Read the model definition and answer for the solid it produces. Units are mm, in the model's axes. Face numbers are marked on the shaded views. Coordinates: 2 decimals unless noted, no trailing zeros. Write each loop counter-clockwise with the first axis right and the second up, starting at its lowest first coordinate (ties: lowest second). Pieces come first, ordered by that corner, then holes. Notation, with made-up numbers: (-32, 34.25) -> (-1, 34.25) arc R24 cw to (-1, 59.25) -> close; hole circle Ø5 at (32.25, 56). An arc over 180 degrees is marked (long way). One line per item, written item: value. Start each with the question number.
1. Consider line 1 along Y through (x, z) = (14.5, 40.5); line 2 along Y through (x, z) = (-51, 8.5); line 3 along X through (y, z) = (-15, 31.5). Determine where each line is inside the solid, lowest interval first.
2. Find section B-B, the plane z = 34.5. Write down the section's boundary in (x, y), and give its area (3 significant figures).
3. Find section C-C, the plane x = -39. Write down the section's boundary in (y, z).
4. Given P1, Ø4, axis at y = -27, z = 23.5, coming from the +X side; P2, Ø9.5, axis at x = -85, y = -45, coming from the +Z side; P3, Ø4, axis at x = -6.5, y = 28.5, coming from the +Z side; P4, Ø4.5, axis at x = 14.47, y = -76.39, coming from the -Z side, each flat-ended and moving along its own axis, determine where each tip first touches the part or whether it passes through.
5. Find section D-D, the plane y = -62.5. Write down the section's boundary in (x, z), and give its area (3 significant figures).
6. For a pull along X with two mould halves and no side action, classify the marked faces 1, 2 and 3 as pulls with the +X half, pulls with the -X half, needs draft (parallel to the pull), parting line crosses it, or undercut.
7. Find section A-A, the plane z = 19. Write down the section's boundary in (x, y).
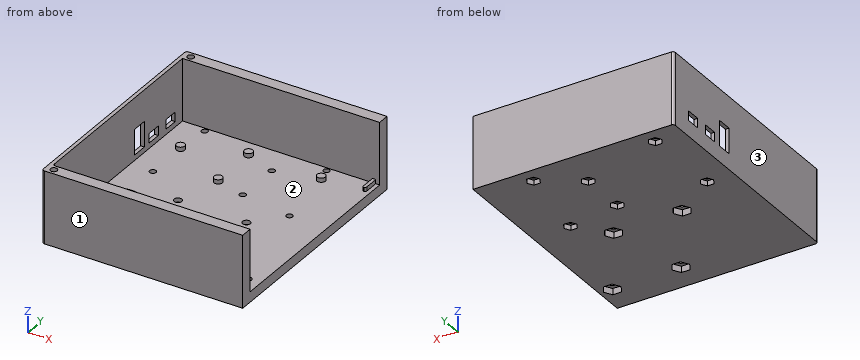
```python
from build123d import *

# Parameters (mm, degrees)
F5_W         = 192.786
F5_H         = 141.3764
F7_DEPTH     = 44.45
F12_W        = 187.452
F12_H        = 127
F14_DEPTH    = 38.1
F4_R         = 15.621
F4_R_2       = 13.081
F13_W        = 2.032
F13_H        = 10.16
F13_W_2      = 10.16
F13_H_2      = 2.032
F15_DEPTH    = 8.89
F16_DEPTH    = 2.9972
F17_DEPTH    = 3.81
F10_R        = 2.3749
F18_DEPTH    = 25.4
F3_R         = 1.9304
F19_DEPTH    = 25.4
F11_R        = 2.54
F20_DEPTH    = 8.89
F21_W        = 8.89
F21_H        = 5.842
F21_W_2      = 9.525
F21_H_2      = 15.621
F22_DEPTH    = 25.4
F23_R        = 2.0828
F24_DEPTH    = 4.318
F25_T1_DEPTH = 41.91
F25_T3_DEPTH = 52.07
F25_T5_DEPTH = 6.35
F26_W        = 69.2167831277
F26_H        = 141.3764
F27_DEPTH    = 50.8


# Not quite as in the source:
# - a fillet or chamfer that OpenCascade refuses, or shapes differently, is made with other operations: its cross-section is extruded or revolved along the edge and cut away or added


with BuildPart() as f7:
    # F5 (on Top) → F7 (new body)
    with BuildSketch(Plane.XY):
        with Locations((-4.773771323, -23.1295908162)):
            Rectangle(F5_W, F5_H)
    extrude(amount=F7_DEPTH)

    # F12 (on face) → F14 (cut)
    with BuildSketch(Plane.XY.offset(44.45)):
        with Locations((-5.154771323, -23.1295908162)):
            Rectangle(F12_W, F12_H)
    extrude(amount=-F14_DEPTH, mode=Mode.SUBTRACT)

    # F4 (on Top) + F13 (on Top) → F15 (join)
    with BuildSketch(Plane.XY):
        with Locations((-81.989771323, -51.9585908162)):
            Circle(F4_R)
        with Locations((-81.989771323, -51.9585908162)):
            Circle(F4_R_2, mode=Mode.SUBTRACT)
    with BuildSketch(Plane.XY):
        with Locations((18.975228677, 35.2904091838)):
            Rectangle(F13_W, F13_H)
        with Locations((47.6495291469, -25.7965908162)):
            Rectangle(F13_W_2, F13_H_2)
    extrude(amount=F15_DEPTH)

    # F6 (on face) → F16 (cut)
    with BuildSketch(Plane.XY):
        Polygon((-81.6243755079, 34.3379091838), (-79.6079796927, 37.8304091838), (-81.6243755079, 41.3229091838), (-85.6571671382, 41.3229091838), (-87.6735629533, 37.8304091838), (-85.6571671382, 34.3379091838), align=None)
        Polygon((-6.6943755079, 34.3379091838), (-4.6779796927, 37.8304091838), (-6.6943755079, 41.3229091838), (-10.7271671382, 41.3229091838), (-12.7435629533, 37.8304091838), (-10.7271671382, 34.3379091838), align=None)
        Polygon((-30.8243755079, 19.0979091838), (-28.8079796927, 22.5904091838), (-30.8243755079, 26.0829091838), (-34.8571671382, 26.0829091838), (-36.8735629533, 22.5904091838), (-34.8571671382, 19.0979091838), align=None)
        Polygon((-82.8943755079, -14.4300908162), (-80.8779796927, -10.9375908162), (-82.8943755079, -7.4450908162), (-86.9271671382, -7.4450908162), (-88.9435629533, -10.9375908162), (-86.9271671382, -14.4300908162), align=None)
        Polygon((-30.8243755079, -9.3500908162), (-28.8079796927, -5.8575908162), (-30.8243755079, -2.3650908162), (-34.8571671382, -2.3650908162), (-36.8735629533, -5.8575908162), (-34.8571671382, -9.3500908162), align=None)
        Polygon((1.1796244921, -14.4300908162), (3.1960203073, -10.9375908162), (1.1796244921, -7.4450908162), (-2.8531671382, -7.4450908162), (-4.8695629533, -10.9375908162), (-2.8531671382, -14.4300908162), align=None)
    extrude(amount=F16_DEPTH, mode=Mode.SUBTRACT)

    # F9 (on Top) → F17 (cut)
    with BuildSketch(Plane.XY):
        Polygon((-55.7338586688, -33.239207965), (-53.0355544507, -28.565607965), (-55.7338586688, -23.892007965), (-61.130467105, -23.892007965), (-63.828771323, -28.565607965), (-61.130467105, -33.239207965), align=None)
        Polygon((-24.9998586688, -81.067407965), (-22.3015544507, -76.393807965), (-24.9998586688, -71.720207965), (-30.396467105, -71.720207965), (-33.094771323, -76.393807965), (-30.396467105, -81.067407965), align=None)
        Polygon((17.1641413312, -71.720207965), (14.4658371131, -71.720207965), (11.767532895, -71.720207965), (9.069228677, -76.393807965), (11.767532895, -81.067407965), (17.1641413312, -81.067407965), (19.8624455493, -76.393807965), align=None)
        Polygon((-10.8715544507, -28.565607965), (-13.5698586688, -23.892007965), (-18.966467105, -23.892007965), (-21.664771323, -28.565607965), (-18.966467105, -33.239207965), (-13.5698586688, -33.239207965), align=None)
    extrude(amount=F17_DEPTH, mode=Mode.SUBTRACT)

    # F10 (on Top) → F18 (cut)
    with BuildSketch(Plane.XY):
        with Locations((-58.4321628869, -28.565607965)):
            Circle(F10_R)
        with Locations((-27.6981628869, -76.393807965)):
            Circle(F10_R)
        with Locations((-16.2681628869, -28.565607965)):
            Circle(F10_R)
        with Locations((14.4658371131, -76.393807965)):
            Circle(F10_R)
    extrude(amount=F18_DEPTH, mode=Mode.SUBTRACT)

    # F3 (on Top) → F19 (cut)
    with BuildSketch(Plane.XY):
        with Locations((-84.910771323, -10.9375908162)):
            Circle(F3_R)
        with Locations((-32.840771323, -5.8575908162)):
            Circle(F3_R)
        with Locations((-32.840771323, 22.5904091838)):
            Circle(F3_R)
        with Locations((-8.710771323, 37.8304091838)):
            Circle(F3_R)
        with Locations((-83.640771323, 37.8304091838)):
            Circle(F3_R)
        with Locations((-0.836771323, -10.9375908162)):
            Circle(F3_R)
    extrude(amount=F19_DEPTH, mode=Mode.SUBTRACT)

    # F11 (on Top) → F20 (join)
    with BuildSketch(Plane.XY):
        with Locations((-6.1370921321, 28.5807047039)):
            Circle(F11_R)
        with Locations((-51.3140404916, 29.3099723562)):
            Circle(F11_R)
        with Locations((-50.6939233637, -1.3771463051)):
            Circle(F11_R)
        with Locations((-84.7697969953, 15.9851294398)):
            Circle(F11_R)
    extrude(amount=F20_DEPTH)

    # F21 (on face) → F22 (cut)
    with BuildSketch(Plane(origin=(-101.166771323, 0, 0), x_dir=(0, -1, 0), z_dir=(-1, 0, 0))):
        with Locations((-12.1256091838, 12.573)):
            Rectangle(F21_W, F21_H)
        with Locations((-28.6356091838, 12.573)):
            Rectangle(F21_W, F21_H)
        with Locations((1.7808908162, 17.4625)):
            Rectangle(F21_W_2, F21_H_2)
    extrude(amount=-F22_DEPTH, mode=Mode.SUBTRACT)

    # F23 (on face) → F24 (cut)
    with BuildSketch(Plane.XY.offset(44.45)):
        with Locations((-96.086771323, -90.2236908162)):
            Circle(F23_R)
        with Locations((86.539228677, -90.2236908162)):
            Circle(F23_R)
        with Locations((86.539228677, 43.9645091838)):
            Circle(F23_R)
        with Locations((-96.086771323, 43.9645091838)):
            Circle(F23_R)
    extrude(amount=-F24_DEPTH, mode=Mode.SUBTRACT)

    # F25: fillet of radius 1.524 on 12 edges, made by hand

    # F25_s2 → F25_t1 (join)
    with BuildSketch(Plane.XY.offset(2.54)):
        with BuildLine():
            ThreePointArc((-97.356771323, -86.6295908162), (-98.4344020576, -86.1832215507), (-98.880771323, -85.1055908162))
            Line((-98.880771323, -85.1055908162), (-98.880771323, -86.6295908162))
            Line((-98.880771323, -86.6295908162), (-97.356771323, -86.6295908162))
        make_face()
        with BuildLine():
            ThreePointArc((88.571228677, -85.1055908162), (88.1248594115, -86.1832215507), (87.047228677, -86.6295908162))
            Line((87.047228677, -86.6295908162), (88.571228677, -86.6295908162))
            Line((88.571228677, -86.6295908162), (88.571228677, -85.1055908162))
        make_face()
    extrude(amount=F25_T1_DEPTH)

    # F25_s4 → F25_t3 (cut)
    with BuildSketch(Plane.XY.offset(-3.81)):
        with BuildLine():
            ThreePointArc((-99.642771323, 47.5586091838), (-100.7204020576, 47.1122399184), (-101.166771323, 46.0346091838))
            Line((-101.166771323, 46.0346091838), (-101.166771323, 47.5586091838))
            Line((-101.166771323, 47.5586091838), (-99.642771323, 47.5586091838))
        make_face()
        with BuildLine():
            ThreePointArc((-101.166771323, -92.2937908162), (-100.7204020576, -93.3714215507), (-99.642771323, -93.8177908162))
            Line((-99.642771323, -93.8177908162), (-101.166771323, -93.8177908162))
            Line((-101.166771323, -93.8177908162), (-101.166771323, -92.2937908162))
        make_face()
        with BuildLine():
            ThreePointArc((91.619228677, -92.2937908162), (91.1728594115, -93.3714215507), (90.095228677, -93.8177908162))
            Line((90.095228677, -93.8177908162), (91.619228677, -93.8177908162))
            Line((91.619228677, -93.8177908162), (91.619228677, -92.2937908162))
        make_face()
        with BuildLine():
            ThreePointArc((90.095228677, 47.5586091838), (91.1728594115, 47.1122399184), (91.619228677, 46.0346091838))
            Line((91.619228677, 46.0346091838), (91.619228677, 47.5586091838))
            Line((91.619228677, 47.5586091838), (90.095228677, 47.5586091838))
        make_face()
    extrude(amount=F25_T3_DEPTH, mode=Mode.SUBTRACT)

    # F25_s6 → F25_t5 (cut)
    with BuildSketch(Plane.XY.offset(6.35)):
        with BuildLine():
            ThreePointArc((17.959228677, 31.7344091838), (18.4055979424, 30.6567784493), (19.483228677, 30.2104091838))
            Line((19.483228677, 30.2104091838), (17.959228677, 30.2104091838))
            Line((17.959228677, 30.2104091838), (17.959228677, 31.7344091838))
        make_face()
        with BuildLine():
            ThreePointArc((42.5695291469, -25.2885908162), (43.0158984124, -26.3662215507), (44.0935291469, -26.8125908162))
            Line((44.0935291469, -26.8125908162), (42.5695291469, -26.8125908162))
            Line((42.5695291469, -26.8125908162), (42.5695291469, -25.2885908162))
        make_face()
        with BuildLine():
            ThreePointArc((42.5695291469, -26.3045908162), (43.0158984124, -25.2269600816), (44.0935291469, -24.7805908162))
            Line((44.0935291469, -24.7805908162), (42.5695291469, -24.7805908162))
            Line((42.5695291469, -24.7805908162), (42.5695291469, -26.3045908162))
        make_face()
        with BuildLine():
            ThreePointArc((19.991228677, 31.7344091838), (19.5448594115, 30.6567784493), (18.467228677, 30.2104091838))
            Line((18.467228677, 30.2104091838), (19.991228677, 30.2104091838))
            Line((19.991228677, 30.2104091838), (19.991228677, 31.7344091838))
        make_face()
        with BuildLine():
            ThreePointArc((51.2055291469, -26.8125908162), (52.2831598814, -26.3662215507), (52.7295291469, -25.2885908162))
            Line((52.7295291469, -25.2885908162), (52.7295291469, -26.8125908162))
            Line((52.7295291469, -26.8125908162), (51.2055291469, -26.8125908162))
        make_face()
        with BuildLine():
            ThreePointArc((51.2055291469, -24.7805908162), (52.2831598814, -25.2269600816), (52.7295291469, -26.3045908162))
            Line((52.7295291469, -26.3045908162), (52.7295291469, -24.7805908162))
            Line((52.7295291469, -24.7805908162), (51.2055291469, -24.7805908162))
        make_face()
    extrude(amount=F25_T5_DEPTH, mode=Mode.SUBTRACT)

    # F26 (on Top) → F27 (cut)
    with BuildSketch(Plane.XY):
        with Locations((57.0108371131, -23.1295908162)):
            Rectangle(F26_W, F26_H)
    extrude(amount=F27_DEPTH, mode=Mode.SUBTRACT)


solid = f7.part
```
Answer block:
1. line 1: y = -93.82 to -86.63, 40.37 to 47.56
1. line 2: y = -93.82 to -86.63, -3.9 to 1.14, 26.79 to 31.83, 40.37 to 47.56
1. line 3: x = -101.17 to -98.88
2. outline: (-101.17, -92.29) arc R1.52 ccw to (-99.64, -93.82) -> (22.4, -93.82) -> (22.4, -86.63) -> (-97.36, -86.63) arc R1.52 cw to (-98.88, -85.11) -> (-98.88, 40.37) -> (22.4, 40.37) -> (22.4, 47.56) -> (-99.64, 47.56) arc R1.52 ccw to (-101.17, 46.03) -> close
2. area: 2,070 mm2
3. outline: (-93.82, 0) -> (47.56, 0) -> (47.56, 44.45) -> (40.37, 44.45) -> (40.37, 6.35) -> (-86.63, 6.35) -> (-86.63, 44.45) -> (-93.82, 44.45) -> close
4. P1: stops at x = -98.88
4. P2: stops at z = 6.35
4. P3: stops at z = 8.89
4. P4: passes through
5. outline: (-101.17, 0) -> (22.4, 0) -> (22.4, 6.35) -> (-70.46, 6.35) -> (-70.46, 8.89) -> (-74.24, 8.89) -> (-74.24, 6.35) -> (-89.74, 6.35) -> (-89.74, 8.89) -> (-93.52, 8.89) -> (-93.52, 6.35) -> (-98.88, 6.35) -> (-98.88, 44.45) -> (-101.17, 44.45) -> close
5. area: 891 mm2
6. face 1: needs draft
6. face 2: undercut
6. face 3: pulls with the -X half
7. outline: (-101.17, -92.29) arc R1.52 ccw to (-99.64, -93.82) -> (22.4, -93.82) -> (22.4, -86.63) -> (-97.36, -86.63) arc R1.52 cw to (-98.88, -85.11) -> (-98.88, -6.54) -> (-101.17, -6.54) -> close; (-101.17, 2.98) -> (-98.88, 2.98) -> (-98.88, 40.37) -> (22.4, 40.37) -> (22.4, 47.56) -> (-99.64, 47.56) arc R1.52 ccw to (-101.17, 46.03) -> close
